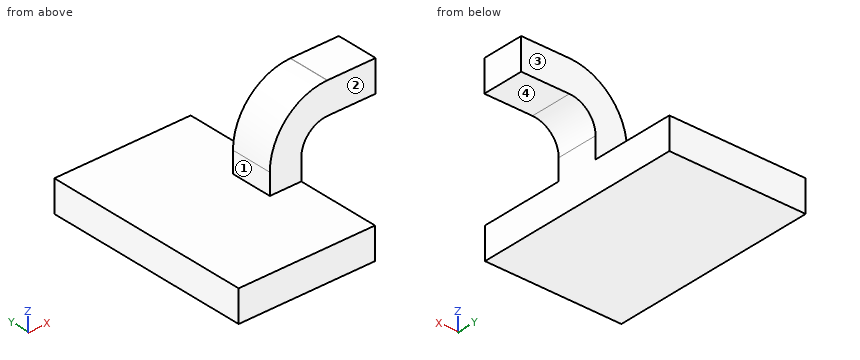
```python
from build123d import *

# Parameters (mm, degrees)
F1_DEPTH = 63.5
F0_W     = 25.0981404377
F0_H     = 19.05
F2_DEPTH = 12.7


# Not quite as in the source:
# - a feature of the source that left no trace in its solid (it failed there, or was rolled back) is left out


with BuildPart() as f1:
    # F0 (on Front) → F1 (new body, symmetric)
    with BuildSketch(Plane.XZ):
        Polygon((-41.275, 9.525), (-41.275, -9.525), (41.275, -9.525), (41.275, 9.525), (22.225, 9.525), align=None)
    extrude(amount=F1_DEPTH, both=True)

    # F0 (on Front) → F2 (join, symmetric)
    with BuildSketch(Plane.XZ):
        with BuildLine():
            Line((22.225, 9.525), (41.275, 9.525))
            Line((41.275, 9.525), (41.275, 22.225))
            ThreePointArc((41.275, 22.225), (45.9246798487, 33.4503201513), (57.15, 38.1))
            Line((57.15, 38.1), (61.2148200089, 38.1))
            Line((61.2148200089, 38.1), (61.2148200089, 57.15))
            Line((61.2148200089, 57.15), (57.15, 57.15))
            add(Edge.make_bspline(
                [(56.9224584332, 57.1492587586), (56.9983070138, 57.1495642251), (57.0741542652, 57.1498113371), (57.15, 57.15)],
                knots=[109.1715172756, 109.1715172756, 109.1715172756, 109.1715172756, 109.3417635215, 109.3417635215, 109.3417635215, 109.3417635215], degree=3))
            ThreePointArc((56.9224584332, 57.1492587586), (32.3739781823, 46.8401247791), (22.225, 22.225))
            Line((22.225, 22.225), (22.225, 9.525))
        make_face()
        with Locations((73.7638902278, 47.625)):
            Rectangle(F0_W, F0_H)
    extrude(amount=F2_DEPTH, both=True)


solid = f1.part
```
Model file for the job. Use its own axes, mm. Face numbers are marked on the shaded views. A direction names the side the tool comes from. Coordinates: 2 decimals unless noted, no trailing zeros. Order: outer loops, then holes, each group sorted by start corner. A loop starts at its lowest first (then second) coordinate and runs counter-clockwise, first axis right, second up. Notation, with made-up numbers: (18, -8) - (59, -8) arc R9 ccw to (59, 8) - close; hole circle Ø11 at (-38, 36). An arc over 180 degrees is marked (long way). Return JSON: item names as keys, results as strings. Group by question number.
1) Tool access for the marked faces 1, 2, 3 and 4: list every direction of +Z, -Z, +X, -X, +Y, -Y with a clear straight run to the whole face (end or side of a thin tool).
2) Saw through at A-A, the plane x = 63. Write the cut outline in (y, z), plus the area to 3 significant figures.
3) Saw through at B-B, the plane z = 3. Write the cut outline in (x, y) (3 decimals).
4) Flat gauge pins, fed straight in: P1, Ø6, axis at x = 64, y = -17, coming from the -Z side; P2, Ø8, axis at x = -17.5, y = -4.5, coming from the +Z side (3 decimals); P3, Ø4, axis at y = -4.5, z = 14.5, coming from the -X side (3 decimals); P4, Ø7.5, axis at x = 68, y = 4, coming from the -Z side. Where does each tip first touch, or does it go through?
5) Probe line 1 (X direction, y = -36, z = 1) (3 decimals); line 2 (Z direction, x = -33, y = 3.5) (3 decimals); line 3 (X direction, y = 9.5, z = 12.5) (3 decimals). List the from-to ranges inside material, lowest first. Write a range as from..to.
Values found:
{
 "1": {"face 1": "+Z, -X, +Y, -Y", "face 2": "+Z, +X, -X, -Y", "face 3": "+Z, +X, -X, +Y", "face 4": "-Z, +X, +Y, -Y"},
 "2": {"outline": "(-12.7, 38.1) - (12.7, 38.1) - (12.7, 57.15) - (-12.7, 57.15) - close", "area": "484 mm²"},
 "3": {"outline": "(-41.275, -63.5) - (41.275, -63.5) - (41.275, 63.5) - (-41.275, 63.5) - close"},
 "4": {"P1": "passes through", "P2": "stops at z = 9.525", "P3": "stops at x = 22.225", "P4": "stops at z = 38.1"},
 "5": {"line 1": "x = -41.275..41.275", "line 2": "z = -9.525..9.525", "line 3": "x = 22.225..41.275"}
}
